Autodesk Inventor part; units mm, degrees
ref_plane "YZ Plane" through (0, 0, 0) normal (1, 0, 0) x (0, 1, 0)
ref_plane "XZ Plane" through (0, 0, 0) normal (0, 1, 0) x (-1, 0, 0)
ref_plane "XY Plane" through (0, 0, 0) normal (0, 0, 1) x (1, 0, 0)
sketch "Sketch1" plane through (0, 0, 0) normal (0, 0, 1) x (1, 0, 0)
  line L0 (-48.4923, 85.7611) -> (-48.4923, 34.9611)
  line L1 (-48.4923, 34.9611) -> (-29.6963, 34.9611)
  line L2 (-29.6963, 34.9611) -> (-29.6963, -41.2389)
  line L3 (-29.6963, -41.2389) -> (986.3037, -41.2389)
  line L4 (986.3037, -41.2389) -> (986.3037, 34.9611)
  line L5 (986.3037, 34.9611) -> (1005.0997, 34.9611)
  line L6 (1005.0997, 34.9611) -> (1005.0997, 85.7611)
  line L7 (1005.0997, 85.7611) -> (986.3037, 85.7611)
  line L8 (986.3037, 85.7611) -> (986.3037, 161.9611)
  line L9 (986.3037, 161.9611) -> (-29.6963, 161.9611)
  line L10 (-48.4923, 85.7611) -> (-29.6963, 85.7611)
  line L11 (-29.6963, 85.7611) -> (-29.6963, 161.9611)
  point P0 (0, 0)
  dimension "d0" = 50.8
  dimension "d1" = 18.796
  dimension "d2" = 76.2
  dimension "d3" = 1016
  dimension "d4" = 76.2
  dimension "d5" = 18.796
  dimension "d6" = 50.8
  dimension "d7" = 76.2
  dimension "d8" = 18.796
extrude "Extrusion1" add sketch "Sketch1" along normal blind 18.796
sketch "Sketch2" plane through (0, 0, 18.796) normal (0, 0, 1) x (1, 0, 0)
  line L0 (-29.6963, 85.7611) -> (-48.4923, 85.7611)
  line L1 (-48.4923, 34.9611) -> (-29.6963, 34.9611)
  line L2 (1005.0997, 34.9611) -> (1005.0997, 85.7611)
  line L3 (-48.4923, 85.7611) -> (-48.4923, 34.9611)
  point P0 (0, 0)
  point P1 (-39.0943, 60.5407)
  point P2 (986.9445, 85.7611)
  point P3 (986.9445, 34.9611)
  point P4 (995.7017, 60.5407)
  dimension "d11" = 9.398
  dimension "d12" = 9.398
hole "Hole1" at (-29.6963, 85.7611, 18.796) at (-29.6963, 34.9611, 18.796) at (-39.0943, 60.5407, 18.796) at (986.9445, 85.7611, 18.796) at (986.9445, 34.9611, 18.796) at (995.7017, 60.5407, 18.796) direction (0, 0, -1) diameter 6.35 end through all
sketch "Sketch3" plane through (0, 0, 18.796) normal (0, 0, 1) x (1, 0, 0)
  line L0 (-29.6963, -41.2389) -> (986.3037, -41.2389)
  line L1 (8.4037, -41.2389) -> (948.2037, -41.2389)
  line L2 (948.2037, -41.2389) -> (948.2037, 85.7611)
  line L3 (910.1037, 123.8611) -> (46.5037, 123.8611)
  line L4 (8.4037, 85.7611) -> (8.4037, -41.2389)
  line L5 (-29.6963, 31.7861) -> (-29.6963, -41.2389)
  line L6 (986.3037, -41.2389) -> (986.3037, 31.8515)
  arc A0 (11.5787, 123.8611) -> (8.4037, 120.6861) centre (11.5787, 120.6861) ccw
  arc A1 (46.5037, 123.8611) -> (8.4037, 85.7611) centre (46.5037, 85.7611) ccw
  arc A2 (948.2037, 85.7611) -> (910.1037, 123.8611) centre (910.1037, 85.7611) ccw
  point P0 (0, 0)
  point P1 (948.2037, 123.8611)
  point P2 (8.4037, 123.8611)
  dimension "d20" = 38.1
  dimension "d21" = 38.1
  dimension "d22" = 939.8
  dimension "d23" = 165.1
  dimension "d24" = 3.175
  dimension "d25" = 38.1
extrude "Extrusion2" cut sketch "Sketch3" against normal blind 25.4
properties part number "bottom" material "Wood (Birch)"
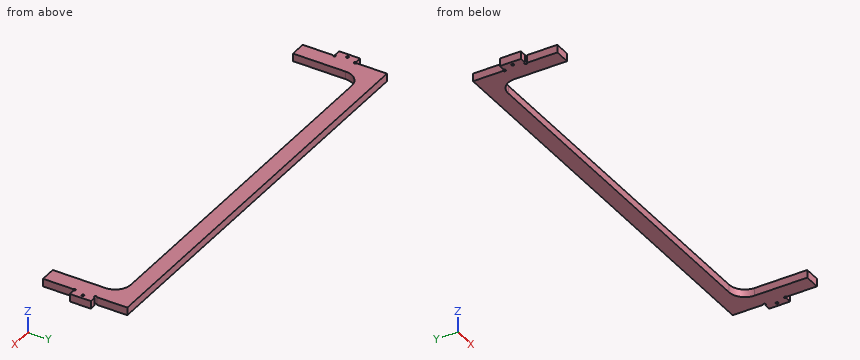
Could you check a few things on this model? Use its own coordinates, in mm. Round coordinates to 2 decimals unless told otherwise and drop trailing zeros. Loops run counter-clockwise (first coordinate to the right, second up) from the corner with the lowest first, then second, coordinate; pieces in that order, holes last. Notation, with made-up numbers: (0, 76) - (5, 76) arc R28 cw to (5, 112) - close; hole circle Ø10 at (17.5, 60.25). An arc over 180 degrees is marked (long way). Answer in a Markdown table with one row per item. Add a question column.
(1) I need wall thicknesses on line 1 along X through (y, z) = (38.5, 13); line 2 along X through (y, z) = (58, 11.25); line 3 along X through (y, z) = (17, 5.25). Which ranges of each line are inside material? Lowest first, please.
(2) If we section it at A-A (y = -22): Please give me the cut outline in (x, z).
(3) If we section it at C-C (x = 358): Please give me the cut outline in (y, z).
(4) If we section it at B-B (z = 5.5): State how many separate pieces and enclosed holes the cut face has, plus the area to 3 significant figures.
(5) I'm going to push flat-ended pins straight in: pin 1 (8.5 mm diameter, centred on x = 995.7, y = 60.54, fed in from -Z); pin 2 (9.5 mm diameter, centred on y = 27.5, z = 11.5, fed in from +X); pin 3 (5 mm diameter, centred on x = -29.7, y = 85.76, fed in from -Z); pin 4 (5.5 mm diameter, centred on x = 608.5, z = 11, fed in from -Y). Where does each tip first touch, or does it pass through?
Model answer:
| question | item | result |
|---|---|---|
| 1 | line 1 | x = -48.49 to 8.4, 948.2 to 1005.1 |
| 1 | line 2 | x = -48.49 to -41, -37.19 to 8.4, 948.2 to 993.8, 997.61 to 1005.1 |
| 1 | line 3 | x = -29.7 to 8.4, 948.2 to 986.3 |
| 2 | outline | (-29.7, 0) - (8.4, 0) - (8.4, 18.8) - (-29.7, 18.8) - close; (948.2, 0) - (986.3, 0) - (986.3, 18.8) - (948.2, 18.8) - close |
| 3 | outline | (123.86, 0) - (161.96, 0) - (161.96, 18.8) - (123.86, 18.8) - close |
| 4 | separate pieces | 1 |
| 4 | enclosed holes | 2 |
| 4 | area | 53,700 mm² |
| 5 | pin 1 | stops at z = 0 |
| 5 | pin 2 | stops at x = 986.3 |
| 5 | pin 3 | passes through |
| 5 | pin 4 | stops at y = 123.86 |
